Design review of the part shown in the three views and the two pictorial views. Dimensions are in mm from the part's minimum x, y and z. A direction names the side the tool comes from. Coordinates: 2 decimals unless noted, no trailing zeros. Write each loop counter-clockwise with the first axis right and the second up, starting at its lowest first coordinate (ties: lowest second). Pieces come first, ordered by that corner, then holes. Notation, with made-up numbers: (-4, -22.75) - (31, -22.75) arc R25 ccw to (31, 16.25) - close; hole circle Ø1 at (60, 64.25). An arc over 180 degrees is marked (long way). Return JSON: item names as keys, results as strings. Group by question number.
(1) We need section D-D on y = 29. State the section outline as (x, z) points.
(2) Draft analysis for pull direction Y (two halves, no side actions). For the marked faces 4, 5 and 6, state which applies: released by +Y, released by -Y, zero draft, split by the parting line, or undercut.
(3) We need section A-A on y = 23. State the section outline as (x, z) points.
(4) Tool access review of the marked faces 1, 2 and 3: name each direction out of +Z, -Z, +X, -X, +Y, -Y from which nothing blocks a thin tool from reaching the whole face with its end or side.
(5) We need section C-C on z = 5. State the section outline as (x, y) points, then the cut area to 3 significant figures.
(6) To check wall thickness, follow L1, parallel to Z at x = 5, y = 26.5; L2, parallel to Z at x = 41, y = 33.25; L3, parallel to Y at x = 20, z = 6.5. State the ranges of each line that lie inside material, in increasing order. Write a range as from..to.
(7) For pin 1 Ø1.5 at (y, z) = (33.5, 3) entering from -X; pin 2 Ø3.5 at (x, z) = (5, 5) entering from -Y; pin 3 Ø1 at (x, z) = (63, 1) entering from -Y; pin 4 Ø3 at (y, z) = (16.5, 6.5) entering from +X, all flat-tipped, find the tip position at first contact; note any pin that passes through.
(8) We need section B-B on x = 41. State the section outline as (y, z) points.
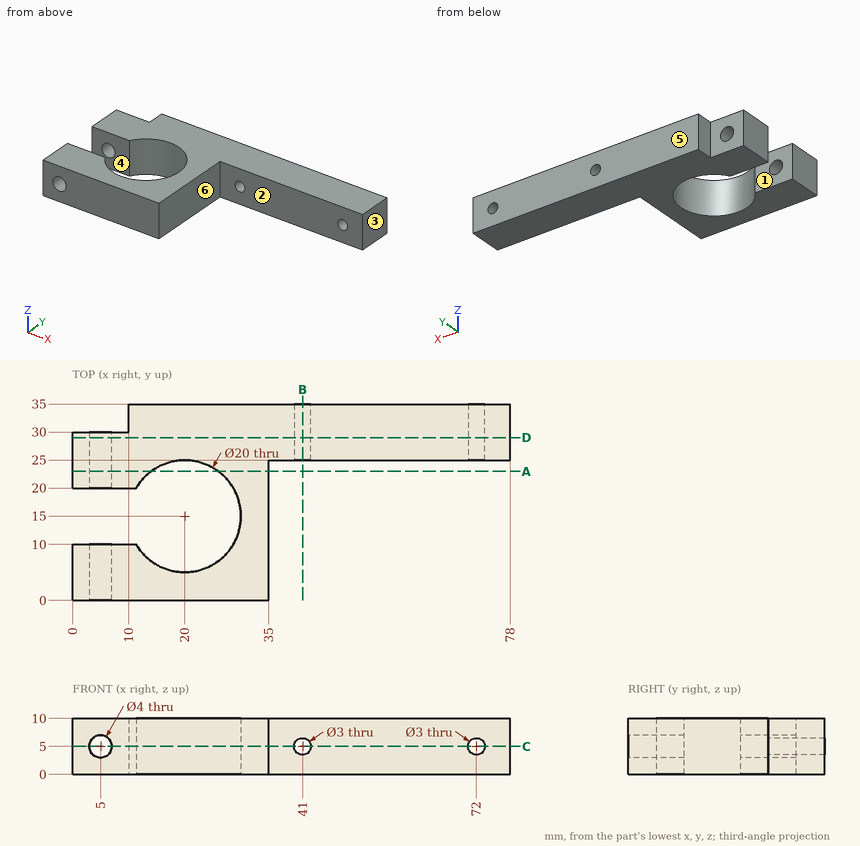
Ans:
{
 "1": {"outline": "(0, 0) - (78, 0) - (78, 10) - (0, 10) - close; hole circle Ø4 at (5, 5); hole circle Ø3 at (41, 5); hole circle Ø3 at (72, 5)"},
 "2": {"face 4": "undercut", "face 5": "released by +Y", "face 6": "zero draft"},
 "3": {"outline": "(0, 0) - (14, 0) - (14, 10) - (0, 10) - close; (26, 0) - (35, 0) - (35, 10) - (26, 10) - close; hole circle Ø4 at (5, 5)"},
 "4": {"face 1": "+Z, -Z, -X", "face 2": "+Z, -Z, +X, -Y", "face 3": "+Z, -Z, +X, +Y, -Y"},
 "5": {"outline": "(0, 0) - (3, 0) - (3, 10) - (0, 10) - close; (0, 20) - (3, 20) - (3, 30) - (0, 30) - close; (7, 0) - (35, 0) - (35, 25) - (39.5, 25) - (39.5, 35) - (10, 35) - (10, 30) - (7, 30) - (7, 20) - (11.34, 20) arc R10 cw (long way) to (11.34, 10) - (7, 10) - close; (42.5, 25) - (70.5, 25) - (70.5, 35) - (42.5, 35) - close; (73.5, 25) - (78, 25) - (78, 35) - (73.5, 35) - close", "area": "1,050 mm²"},
 "6": {"L1": "0..3, 7..10", "L2": "0..3.5, 6.5..10", "L3": "0..5, 25..35"},
 "7": {"pin 1": "x = 10", "pin 2": "through", "pin 3": "y = 25", "pin 4": "x = 35"},
 "8": {"outline": "(25, 0) - (35, 0) - (35, 3.5) - (25, 3.5) - close; (25, 6.5) - (35, 6.5) - (35, 10) - (25, 10) - close"}
}
